Here's how the part is built. I have some questions about the finished solid (model axes, mm). A direction names the side the tool comes from. Coordinates: 2 decimals unless noted, no trailing zeros. Order: outer loops, then holes, each group sorted by start corner. A loop starts at its lowest first (then second) coordinate and runs counter-clockwise, first axis right, second up. Notation, with made-up numbers: (-15, 33) - (36, 33) arc R30 cw to (36, 72) - close; hole circle Ø11 at (32, -35.5). An arc over 180 degrees is marked (long way). Answer as CSV lines item,"result". Start each with the question number.
Q1. Thinking about a two-plate mould opening in X: for faces 3 (the face through (21, 0, -69)), 4 (the face through (32.747, 7.383, -10.121)), 5 (the face through (0, 7, -36)), which applies, released by +X, released by -X, zero draft, split by the parting line, or undercut?
Q2. For faces 1 (the face through (60, 7, -92)), 2 (the face through (40, 7, -36)), which set-ups out of +Z, -Z, +X, -X, +Y, -Y let a thin tool reach every point of the face, with its end or its side?
Q3. Suppose I cut it at C-C (z = -20). Please give me the cut outline in (x, y).
Q4. I need wall thicknesses on line 1 (Z direction, x = 30, y = 11); line 2 (X direction, y = 5.75, z = -30); line 3 (Z direction, x = 28.5, y = 10). Which ranges of each line are inside material? Lowest first, please.
Q5. Suppose I cut it at A-A (z = -92.15). Please give me the cut outline in (x, y) (3 decimals), then the cut area to 4 significant figures.
Q6. Suppose I cut it at B-B (y = 3.25). Count the separate pieces of the cut face and the enclosed holes in it, then the cut area to 3 significant figures.
Q7. For pin 1 Ø4 at (x, y) = (-10, 3) entering from +Z; pin 2 Ø1 at (y, z) = (4, -19) entering from +X; pin 3 Ø7 at (x, z) = (10, -30) entering from -Y; pin 4 Ø4.5 at (y, z) = (9.5, -43) entering from -X, each with a flat end and sliding along its axis, tell me the tip position at first contact or that it passes through.
from build123d import *

# Parameters (mm, degrees)
BOSS_EXTRUDE1_DEPTH            = 15
M5_CLEARANCE_HOLE1_D           = 5.5
M5_CLEARANCE_HOLE1_CSINK_D     = 5.55
M5_CLEARANCE_HOLE1_CSINK_ANGLE = 90
FILLET1_START                  = -1
FILLET1_DEPTH                  = 17
FILLET1_2_DEPTH                = 15


with BuildPart() as part:
    # Sketch1 → Boss-Extrude1 (new body)
    with BuildSketch(Plane(origin=(0, 0, 0), x_dir=(1, 0, 0), z_dir=(0, 1, 0))):
        Polygon((0, 0), (40, 0), (40, 72.15), (60, 72.15), (60, 112.15), (-20, 112.15), (-20, 72.15), (0, 72.15), align=None)
    extrude(amount=BOSS_EXTRUDE1_DEPTH)

    # M5 Clearance Hole1 (through all)
    with Locations(Plane(origin=(0, 15, 0), x_dir=(1, 0, 0), z_dir=(0, 1, 0))):
        with Locations((-1.85, 92.15), (41.85, 92.15), (10, 30), (30, 30), (10, 10), (30, 10)):
            CounterSinkHole(M5_CLEARANCE_HOLE1_D / 2, M5_CLEARANCE_HOLE1_CSINK_D / 2, counter_sink_angle=M5_CLEARANCE_HOLE1_CSINK_ANGLE)

    # Fillet1: read off the stored shape, not the designer's step
    # Fillet1 outline → Fillet1 (cut)
    with BuildSketch(Plane(origin=(0, 0, 0), x_dir=(1, 0, 0), z_dir=(0, 1, 0)).offset(FILLET1_START)):
        with BuildLine():
            Line((0, 0), (10, 0))
            add(Edge.make_bspline(
                [(10, 0), (0, 0), (0, 10)],
                knots=[0, 0, 0, 1, 1, 1], degree=2, weights=[1, 0.707106781, 1]))
            Line((0, 10), (0, 0))
        make_face()
        with BuildLine():
            add(Edge.make_bspline(
                [(40, 10), (40, 0), (30, 0)],
                knots=[0, 0, 0, 1, 1, 1], degree=2, weights=[1, 0.707106781, 1]))
            Line((30, 0), (40, 0))
            Line((40, 0), (40, 10))
        make_face()
        with BuildLine():
            Line((-20, 72.15), (-10, 72.15))
            add(Edge.make_bspline(
                [(-10, 72.15), (-20, 72.15), (-20, 82.15)],
                knots=[0, 0, 0, 1, 1, 1], degree=2, weights=[1, 0.707106781, 1]))
            Line((-20, 82.15), (-20, 72.15))
        make_face()
        with BuildLine():
            add(Edge.make_bspline(
                [(60, 82.15), (60, 72.15), (50, 72.15)],
                knots=[0, 0, 0, 1, 1, 1], degree=2, weights=[1, 0.707106781, 1]))
            Line((50, 72.15), (60, 72.15))
            Line((60, 72.15), (60, 82.15))
        make_face()
        with BuildLine():
            Line((-20, 112.15), (-20, 102.15))
            add(Edge.make_bspline(
                [(-20, 102.15), (-20, 112.15), (-10, 112.15)],
                knots=[0, 0, 0, 1, 1, 1], degree=2, weights=[1, 0.707106781, 1]))
            Line((-10, 112.15), (-20, 112.15))
        make_face()
        with BuildLine():
            add(Edge.make_bspline(
                [(50, 112.15), (60, 112.15), (60, 102.15)],
                knots=[0, 0, 0, 1, 1, 1], degree=2, weights=[1, 0.707106781, 1]))
            Line((60, 102.15), (60, 112.15))
            Line((60, 112.15), (50, 112.15))
        make_face()
    extrude(amount=FILLET1_DEPTH, mode=Mode.SUBTRACT)

    # Fillet1 2 outline → Fillet1 2 (add)
    with BuildSketch(Plane(origin=(0, 0, 0), x_dir=(1, 0, 0), z_dir=(0, 1, 0))):
        with BuildLine():
            add(Edge.make_bspline(
                [(0, 62.15), (0, 72.15), (-10, 72.15)],
                knots=[0, 0, 0, 1, 1, 1], degree=2, weights=[1, 0.707106781, 1]))
            Line((0, 62.15), (0, 72.15))
            Line((0, 72.15), (-10, 72.15))
        make_face()
        with BuildLine():
            Line((40, 72.15), (40, 62.15))
            add(Edge.make_bspline(
                [(50, 72.15), (40, 72.15), (40, 62.15)],
                knots=[0, 0, 0, 1, 1, 1], degree=2, weights=[1, 0.707106781, 1]))
            Line((50, 72.15), (40, 72.15))
        make_face()
    extrude(amount=FILLET1_2_DEPTH)


solid = part.part
Here are the results:
1,face 3,"zero draft"
1,face 4,"undercut"
1,face 5,"released by -X"
2,face 1,"+Z, -Z, +X, +Y, -Y"
2,face 2,"+Z, +X, +Y, -Y"
3,outline,"(0, 0) - (40, 0) - (40, 15) - (0, 15) - close"
4,line 1,"z = -112.15 to -32.75, -27.25 to -12.75, -7.25 to 0"
4,line 2,"x = 0 to 7.25, 12.75 to 27.25, 32.75 to 40"
4,line 3,"z = -112.15 to -32.3, -27.7 to -12.3, -7.7 to 0"
5,outline,"(-20, 0) - (-4.6, 0) - (-4.6, 14.975) - (-4.625, 15) - (-20, 15) - close; (0.9, 0) - (39.1, 0) - (39.1, 14.975) - (39.075, 15) - (0.925, 15) - (0.9, 14.975) - close; (44.6, 0) - (60, 0) - (60, 15) - (44.625, 15) - (44.6, 14.975) - close"
5,area,"1,035 mm²"
6,separate pieces,"1"
6,enclosed holes,"6"
6,area,"5,860 mm²"
7,pin 1,"stops at z = -71.95"
7,pin 2,"stops at x = 40"
7,pin 3,"stops at y = 0"
7,pin 4,"stops at x = 0"
